```python
from build123d import *

# Parameters (mm, degrees)
CROQUIS1_R              = 44.45
CROQUIS1_R_2            = 38.95
SALIENTE_EXTRUIR1_DEPTH = 1144
CORTAR_EXTRUIR1_START   = -101.6
CORTAR_EXTRUIR1_DEPTH   = 101.6


with BuildPart() as part:
    # Croquis1 → Saliente-Extruir1 (new body)
    with BuildSketch(Plane(origin=(0, 0, 0), x_dir=(0, 0, -1), z_dir=(1, 0, 0))):
        Circle(CROQUIS1_R)
        Circle(CROQUIS1_R_2, mode=Mode.SUBTRACT)
    extrude(amount=SALIENTE_EXTRUIR1_DEPTH)

    # Croquis3 → Cortar-Extruir1 (cut)
    with BuildSketch(Plane(origin=(1144, 0, 0), x_dir=(0, 0, -1), z_dir=(1, 0, 0)).offset(CORTAR_EXTRUIR1_START)):
        with BuildLine():
            Line((-44.45, 0), (-38.95, 0))
            ThreePointArc((-38.95, 0), (0, -38.95), (38.95, 0))
            Line((38.95, 0), (44.45, 0))
            ThreePointArc((44.45, 0), (0, -44.45), (-44.45, 0))
        make_face()
    extrude(amount=CORTAR_EXTRUIR1_DEPTH, mode=Mode.SUBTRACT)


solid = part.part
```
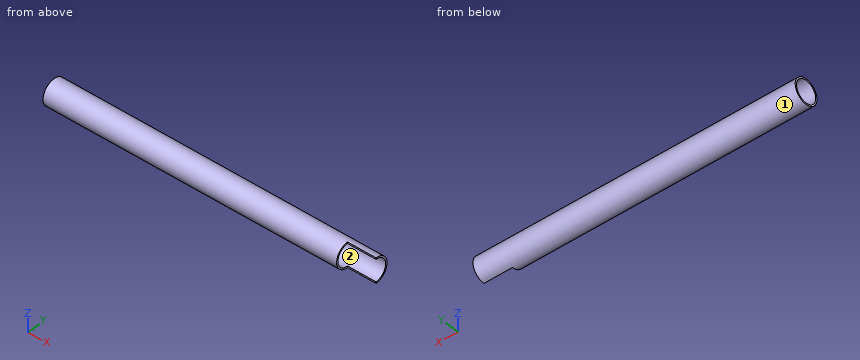
Geometry check sheet. Reference: the model listing, model coordinates, mm. Face numbers are marked on the shaded views. Round coordinates to 2 decimals unless told otherwise and drop trailing zeros. Loops run counter-clockwise (first coordinate to the right, second up) from the corner with the lowest first, then second, coordinate; pieces in that order, holes last. Notation, with made-up numbers: (43, 55.25) - (81, 55.25) arc R10 cw to (81, 60.25) - close; hole circle Ø2 at (73.25, 36.5). An arc over 180 degrees is marked (long way). Write item = value, one per line. Start each with the question number.
1. Thickness scan on line 1 (Y direction, x = 854, z = 0); line 2 (Z direction, x = 286.5, y = -2); line 3 (Z direction, x = 667.5, y = 34). Record the ranges inside material, lowest first.
2. Depth check by flat-ended pin: pin 1 (8 mm diameter, centred on x = 203.5, y = -21.5, fed in from -Z); pin 2 (4.5 mm diameter, centred on x = 1081, z = -40.5, fed in from -Y); pin 3 (8 mm diameter, centred on x = 1004.5, z = 26.5, fed in from -Y). Enter the tip coordinate at first touch or a pass-through.
3. Mould release check, pull along Z, two halves, no side actions. Record for the marked faces 1 and 2: released by +Z, released by -Z, zero draft, split by the parting line, or undercut.
4. Section check B-B on x = 447. Enter the section's corners in (y, z).
5. Section check A-A on z = 0. Enter the section's corners in (x, y).
Working result:
q1.line_1 = -44.45 to -38.95, 38.95 to 44.45
q1.line_2 = -44.4 to -38.9, 38.9 to 44.4
q1.line_3 = -28.63 to -19, 19 to 28.63
q2.pin_1 = -40.86
q2.pin_2 = 0
q2.pin_3 = -38.33
q3.face_1 = split by the parting line
q3.face_2 = undercut
q4.outline = circle Ø88.9 at (0, 0); hole circle Ø77.9 at (0, 0)
q5.outline = (0, -44.45) - (1042.4, -44.45) - (1042.4, -38.95) - (0, -38.95) - close; (0, 38.95) - (1144, 38.95) - (1144, 44.45) - (0, 44.45) - close
